The listing builds one solid part. Answer for the finished solid, in the listing's coordinates (mm). Give positions to 0.01 mm unless a question says otherwise; leave off trailing zeros.
```python
from build123d import *

# Parameters (mm, degrees)
F0_R          = 10.75
F0_R_2        = 4.1
F0_R_3        = 2.5
F1_DEPTH      = 9.6
F2_R          = 8
F3_DEPTH      = 25
F4_DEPTH      = 6.1
F4_DEPTH_BACK = 13.5


with BuildPart() as f1:
    # F0 (on Top) → F1 (new body)
    with BuildSketch(Plane.XY):
        Circle(F0_R)
        Circle(F0_R_2, mode=Mode.SUBTRACT)
        Circle(F0_R_2)
        Circle(F0_R_3, mode=Mode.SUBTRACT)
    extrude(amount=F1_DEPTH)

    # F2
    f2_edges = [f1.edges().sort_by_distance(p)[0] for p in [
        (-10.75, 0, 9.6),
    ]]
    fillet(f2_edges, radius=F2_R)

    # F0 (on Top) → F3 (cut)
    with BuildSketch(Plane.XY):
        Circle(F0_R_3)
    extrude(amount=-F3_DEPTH, mode=Mode.SUBTRACT)

    # F0 (on Top) → F4 (cut, two sides)
    with BuildSketch(Plane.XY) as f4_sk:
        Circle(F0_R_2)
        Circle(F0_R_3, mode=Mode.SUBTRACT)
    extrude(amount=F4_DEPTH, mode=Mode.SUBTRACT)
    extrude(f4_sk.sketch, amount=-F4_DEPTH_BACK, mode=Mode.SUBTRACT)


solid = f1.part
```
Item 1: Consider probe 1 along Z at (x, y) = (-2.5, 1.75); probe 2 along Y at (x, z) = (-1.5, 6.5); probe 3 along X at (y, z) = (-0.75, 7.75). Determine where each line is inside the solid, lowest interval first.
Conclusion:
probe 1: z = 6.1 to 9.59
probe 2: y = -8.95 to -2, 2 to 8.95
probe 3: x = -7.83 to -2.38, 2.38 to 7.83
Item 2: Each of these flat-tipped pins is pushed along its axis until it touches: P1, Ø2.5, axis at x = 1, y = 1.5, coming from the -Z side; P2, Ø2, axis at x = -4, y = -7, coming from the +Z side; P3, Ø5, axis at y = -1.5, z = 1, coming from the +X side; P4, Ø3, axis at x = 3, z = 6.5, coming from the -Y side. Where does it stop, or does it pass through?
Conclusion:
P1: stops at z = 6.1
P2: stops at z = 8.34
P3: stops at x = 10.75
P4: stops at y = -9.64
Item 3: Determine the mould class of faces 1 (the face through (5, 0, 0)), 2 (the face through (-0.534, 4.065, 3.007)), 3 (the face through (-1.4, 10.66, 0.79)), 4 (the face through (-2, -2, 6.1)) for opening direction Y: pulls with the +Y half, pulls with the -Y half, needs draft (parallel to the pull), parting line crosses it, or undercut.
Conclusion:
face 1: needs draft
face 2: undercut
face 3: parting line crosses it
face 4: undercut
